For this review, take the finished solid that the model builds, in its own axes (mm). A direction names the side the tool comes from. Round coordinates to 2 decimals unless told otherwise and drop trailing zeros. Write each loop counter-clockwise with the first axis right and the second up, starting at its lowest first coordinate (ties: lowest second). Pieces come first, ordered by that corner, then holes.
from build123d import *

# Parameters (mm, degrees)
SKETCH1_W           = 80
SKETCH1_H           = 60
BOSS_EXTRUDE1_DEPTH = 10
SKETCH2_W           = 80
SKETCH2_H           = 130
BOSS_EXTRUDE2_DEPTH = 10
CUT_EXTRUDE1_REACH  = 132
SKETCH3_R           = 2.75
CUT_EXTRUDE2_REACH  = 138.015
SKETCH4_R           = 2.75
SKETCH5_W           = 10
SKETCH5_H           = 50
BOSS_EXTRUDE3_DEPTH = 120
CUT_EXTRUDE3_REACH  = 133.624
FILLET1_R           = 10
FILLET2_R           = 3
FILLET3_R           = 3


with BuildPart() as part:
    # Sketch1 → Boss-Extrude1 (new body)
    with BuildSketch(Plane.XY):
        Rectangle(SKETCH1_W, SKETCH1_H)
    extrude(amount=BOSS_EXTRUDE1_DEPTH)

    # Sketch2 → Boss-Extrude2 (add)
    with BuildSketch(Plane(origin=(0, 30, 0), x_dir=(1, 0, 0), z_dir=(0, 1, 0))):
        with Locations((0, 55)):
            Rectangle(SKETCH2_W, SKETCH2_H)
    extrude(amount=-BOSS_EXTRUDE2_DEPTH)

    # Sketch3 → Cut-Extrude1 (cut, up to next)
    with BuildSketch(Plane(origin=(0, 0, 0), x_dir=(-1, 0, 0), z_dir=(0, 0, -1)), mode=Mode.PRIVATE) as cut_extrude1_sk1:
        with Locations((-25, -16.5)):
            Circle(SKETCH3_R)
    cut_extrude1_tool1 = extrude(cut_extrude1_sk1.sketch, amount=-CUT_EXTRUDE1_REACH, mode=Mode.PRIVATE) & part.part
    # Sketch3 → Cut-Extrude1 (cut, up to next)
    with BuildSketch(Plane(origin=(0, 0, 0), x_dir=(-1, 0, 0), z_dir=(0, 0, -1)), mode=Mode.PRIVATE) as cut_extrude1_sk2:
        with Locations((25, -16.5)):
            Circle(SKETCH3_R)
    cut_extrude1_tool2 = extrude(cut_extrude1_sk2.sketch, amount=-CUT_EXTRUDE1_REACH, mode=Mode.PRIVATE) & part.part
    # Sketch3 → Cut-Extrude1 (cut, up to next)
    with BuildSketch(Plane(origin=(0, 0, 0), x_dir=(-1, 0, 0), z_dir=(0, 0, -1)), mode=Mode.PRIVATE) as cut_extrude1_sk3:
        with Locations((-25, -6.5)):
            Circle(SKETCH3_R)
    cut_extrude1_tool3 = extrude(cut_extrude1_sk3.sketch, amount=-CUT_EXTRUDE1_REACH, mode=Mode.PRIVATE) & part.part
    # Sketch3 → Cut-Extrude1 (cut, up to next)
    with BuildSketch(Plane(origin=(0, 0, 0), x_dir=(-1, 0, 0), z_dir=(0, 0, -1)), mode=Mode.PRIVATE) as cut_extrude1_sk4:
        with Locations((25, -6.5)):
            Circle(SKETCH3_R)
    cut_extrude1_tool4 = extrude(cut_extrude1_sk4.sketch, amount=-CUT_EXTRUDE1_REACH, mode=Mode.PRIVATE) & part.part
    # Sketch3 → Cut-Extrude1 (cut, up to next)
    with BuildSketch(Plane(origin=(0, 0, 0), x_dir=(-1, 0, 0), z_dir=(0, 0, -1)), mode=Mode.PRIVATE) as cut_extrude1_sk5:
        with Locations((-25, 3.5)):
            Circle(SKETCH3_R)
    cut_extrude1_tool5 = extrude(cut_extrude1_sk5.sketch, amount=-CUT_EXTRUDE1_REACH, mode=Mode.PRIVATE) & part.part
    # Sketch3 → Cut-Extrude1 (cut, up to next)
    with BuildSketch(Plane(origin=(0, 0, 0), x_dir=(-1, 0, 0), z_dir=(0, 0, -1)), mode=Mode.PRIVATE) as cut_extrude1_sk6:
        with Locations((25, 3.5)):
            Circle(SKETCH3_R)
    cut_extrude1_tool6 = extrude(cut_extrude1_sk6.sketch, amount=-CUT_EXTRUDE1_REACH, mode=Mode.PRIVATE) & part.part
    add(cut_extrude1_tool1.solids().sort_by_distance((25, -16.5, 0))[0], mode=Mode.SUBTRACT)
    add(cut_extrude1_tool2.solids().sort_by_distance((-25, -16.5, 0))[0], mode=Mode.SUBTRACT)
    add(cut_extrude1_tool3.solids().sort_by_distance((25, -6.5, 0))[0], mode=Mode.SUBTRACT)
    add(cut_extrude1_tool4.solids().sort_by_distance((-25, -6.5, 0))[0], mode=Mode.SUBTRACT)
    add(cut_extrude1_tool5.solids().sort_by_distance((25, 3.5, 0))[0], mode=Mode.SUBTRACT)
    add(cut_extrude1_tool6.solids().sort_by_distance((-25, 3.5, 0))[0], mode=Mode.SUBTRACT)

    # Sketch4 → Cut-Extrude2 (cut, up to next)
    with BuildSketch(Plane.XZ.offset(-20), mode=Mode.PRIVATE) as cut_extrude2_sk1:
        with Locations(Location((-32.5, -110, 0), (0, 0, 270))):
            Circle(SKETCH4_R)
    cut_extrude2_tool1 = extrude(cut_extrude2_sk1.sketch, amount=-CUT_EXTRUDE2_REACH, mode=Mode.PRIVATE) & part.part
    # Sketch4 → Cut-Extrude2 (cut, up to next)
    with BuildSketch(Plane.XZ.offset(-20), mode=Mode.PRIVATE) as cut_extrude2_sk2:
        with Locations(Location((32.5, -110, 0), (0, 0, 270))):
            Circle(SKETCH4_R)
    cut_extrude2_tool2 = extrude(cut_extrude2_sk2.sketch, amount=-CUT_EXTRUDE2_REACH, mode=Mode.PRIVATE) & part.part
    # Sketch4 → Cut-Extrude2 (cut, up to next)
    with BuildSketch(Plane.XZ.offset(-20), mode=Mode.PRIVATE) as cut_extrude2_sk3:
        with Locations(Location((-32.5, -70, 0), (0, 0, 270))):
            Circle(SKETCH4_R)
    cut_extrude2_tool3 = extrude(cut_extrude2_sk3.sketch, amount=-CUT_EXTRUDE2_REACH, mode=Mode.PRIVATE) & part.part
    # Sketch4 → Cut-Extrude2 (cut, up to next)
    with BuildSketch(Plane.XZ.offset(-20), mode=Mode.PRIVATE) as cut_extrude2_sk4:
        with Locations(Location((32.5, -70, 0), (0, 0, 270))):
            Circle(SKETCH4_R)
    cut_extrude2_tool4 = extrude(cut_extrude2_sk4.sketch, amount=-CUT_EXTRUDE2_REACH, mode=Mode.PRIVATE) & part.part
    # Sketch4 → Cut-Extrude2 (cut, up to next)
    with BuildSketch(Plane.XZ.offset(-20), mode=Mode.PRIVATE) as cut_extrude2_sk5:
        with Locations(Location((-32.5, -30, 0), (0, 0, 270))):
            Circle(SKETCH4_R)
    cut_extrude2_tool5 = extrude(cut_extrude2_sk5.sketch, amount=-CUT_EXTRUDE2_REACH, mode=Mode.PRIVATE) & part.part
    # Sketch4 → Cut-Extrude2 (cut, up to next)
    with BuildSketch(Plane.XZ.offset(-20), mode=Mode.PRIVATE) as cut_extrude2_sk6:
        with Locations(Location((32.5, -30, 0), (0, 0, 270))):
            Circle(SKETCH4_R)
    cut_extrude2_tool6 = extrude(cut_extrude2_sk6.sketch, amount=-CUT_EXTRUDE2_REACH, mode=Mode.PRIVATE) & part.part
    add(cut_extrude2_tool1.solids().sort_by_distance((-32.5, 20, -110))[0], mode=Mode.SUBTRACT)
    add(cut_extrude2_tool2.solids().sort_by_distance((32.5, 20, -110))[0], mode=Mode.SUBTRACT)
    add(cut_extrude2_tool3.solids().sort_by_distance((-32.5, 20, -70))[0], mode=Mode.SUBTRACT)
    add(cut_extrude2_tool4.solids().sort_by_distance((32.5, 20, -70))[0], mode=Mode.SUBTRACT)
    add(cut_extrude2_tool5.solids().sort_by_distance((-32.5, 20, -30))[0], mode=Mode.SUBTRACT)
    add(cut_extrude2_tool6.solids().sort_by_distance((32.5, 20, -30))[0], mode=Mode.SUBTRACT)

    # Sketch5 → Boss-Extrude3 (add)
    with BuildSketch(Plane(origin=(0, 0, 0), x_dir=(-1, 0, 0), z_dir=(0, 0, -1))):
        with Locations((0, -5)):
            Rectangle(SKETCH5_W, SKETCH5_H)
    extrude(amount=BOSS_EXTRUDE3_DEPTH)

    # Sketch6 → Cut-Extrude3 (cut, up to next)
    with BuildSketch(Plane.ZY.offset(5), mode=Mode.PRIVATE) as cut_extrude3_sk1:
        Polygon((-120, 20), (-120, -30), (0, -30), align=None)
    cut_extrude3_tool1 = extrude(cut_extrude3_sk1.sketch, amount=-CUT_EXTRUDE3_REACH, mode=Mode.PRIVATE) & part.part
    add(cut_extrude3_tool1.solids().sort_by_distance((-5, -13.333333, -80))[0], mode=Mode.SUBTRACT)

    # Fillet1
    fillet1_edges = [part.edges().sort_by_distance(p)[0] for p in [
        (40, 25, -120),
        (-40, 25, -120),
        (40, -30, 5),
        (-40, -30, 5),
    ]]
    fillet(fillet1_edges, radius=FILLET1_R)

    # Fillet2
    fillet2_edges = [part.edges().sort_by_distance(p)[0] for p in [
        (0, 30, 10),
    ]]
    fillet(fillet2_edges, radius=FILLET2_R)

    # Fillet3
    fillet3_edges = [part.edges().sort_by_distance(p)[0] for p in [
        (22.5, 20, 0),
        (-22.5, 20, 0),
        (-5, -5, 0),
        (-5, 20, -60),
        (5, 20, -60),
        (5, -5, 0),
    ]]
    fillet(fillet3_edges, radius=FILLET3_R)


solid = part.part
(1) We need section C-C, the plane z = -30. Give the boundary of the cut face in (x, y).
Geometry check:
outline: (-40, 20) - (-35.25, 20) - (-35.25, 30) - (-40, 30) - close; (-29.75, 20) - (-8, 20) arc R3 cw to (-5, 17) - (-5, -17.5) - (5, -17.5) - (5, 17) arc R3 cw to (8, 20) - (29.75, 20) - (29.75, 30) - (-29.75, 30) - close; (35.25, 20) - (40, 20) - (40, 30) - (35.25, 30) - close
(2) For line 1 along Y through (x, z) = (25, 7); line 2 along X through (y, z) = (25.25, -110); line 3 along Z through (x, y) = (32, 23), list the stretches that pass through material, from the lowest coordinate up.
Geometry check:
line 1: y = -30 to -19.25, -13.75 to -9.25, -3.75 to 0.75, 6.25 to 30
line 2: x = -40 to -35.25, -29.75 to 29.75, 35.25 to 40
line 3: z = -119.8 to -112.7, -107.3 to -72.7, -67.3 to -32.7, -27.3 to 10
(3) For pin 1 Ø9 at (x, y) = (25, 3.5) entering from +Z; pin 2 Ø9 at (x, y) = (-25, -16.5) entering from -Z; pin 3 Ø13.5 at (y, z) = (4, -33) entering from +X; pin 4 Ø5 at (x, z) = (-32.5, -30) entering from -Y, all flat-tipped, find the tip position at first contact; note any pin that passes through.
Geometry check:
pin 1: stops at z = 10
pin 2: stops at z = 0
pin 3: stops at x = 5
pin 4: passes through
(4) We need section A-A, the plane y = 3.5. Give the boundary of the cut face in (x, z), and give its area (3 significant figures).
Geometry check:
outline: (-40, 0) - (-27.75, 0) - (-27.75, 10) - (-40, 10) - close; (-22.25, 0) - (-8, 0) arc R3 cw to (-5, -3) - (-5, -80.4) - (5, -80.4) - (5, -3) arc R3 cw to (8, 0) - (22.25, 0) - (22.25, 10) - (-22.25, 10) - close; (27.75, 0) - (40, 0) - (40, 10) - (27.75, 10) - close
area: 1,500 mm2
(5) Mouldability with a two-part tool opening along X and no side actions: class faces 1 (the face through (-24.22, 19.14, -0.9)), 2 (the face through (-30.641, 24.93, -107.973)), 3 (the face through (5.9, 19.14, -62.32)), 4 (the face through (-5.9, 19.14, -62.32)) as pulls with the +X half, pulls with the -X half, needs draft (parallel to the pull), parting line crosses it, or undercut.
Geometry check:
face 1: needs draft
face 2: undercut
face 3: pulls with the +X half
face 4: pulls with the -X half
(6) We need section D-D, the plane x = -16.5. Give the boundary of the cut face in (y, z), and give its area (3 significant figures).
Geometry check:
outline: (-30, 0) - (17, 0) arc R3 cw to (20, -3) - (20, -120) - (30, -120) - (30, 7) arc R3 ccw to (27, 10) - (-30, 10) - close
area: 1,800 mm2
(7) We need section B-B, the plane x = -25. Give the boundary of the cut face in (y, z).
Geometry check:
outline: (-30, 0) - (-19.25, 0) - (-19.25, 10) - (-30, 10) - close; (-13.75, 0) - (-9.25, 0) - (-9.25, 10) - (-13.75, 10) - close; (-3.75, 0) - (0.75, 0) - (0.75, 10) - (-3.75, 10) - close; (6.25, 0) - (17, 0) arc R3 cw to (20, -3) - (20, -120) - (30, -120) - (30, 7) arc R3 ccw to (27, 10) - (6.25, 10) - close
(8) For faces 5 (the face through (-5, 4, -33)), 6 (the face through (-22.253, 3.621, 4.93)), 7 (the face through (24, 20, -62)), list the 3-axis set-ups (+Z, -Z, +X, -X, +Y, -Y) from which the entire face can be reached by the end or side of a thin tool; tool diameter is ignored.
Geometry check:
face 5: -Z, -X, -Y
face 6: +Z, -Z
face 7: -Z, +X, -Y
